Check sheet for the modelled part. Datum: model origin and axes. Units: mm. Round coordinates to 2 decimals unless told otherwise and drop trailing zeros. Write each loop counter-clockwise with the first axis right and the second up, starting at its lowest first coordinate (ties: lowest second). Pieces come first, ordered by that corner, then holes.
Item 1: Cross-section at D-D on x = 32. Enter the section's corners in (y, z).
Item 2: Cross-section at B-B on z = 1.2. Enter the section's corners in (x, y), plus the area to 3 significant figures.
Item 3: Cross-section at C-C on y = 20.5. Count the separate pieces of the cut face and the enclosed holes in it, plus the area to 3 significant figures.
Item 4: Material ranges on line 1 (X direction, y = 23, z = 0.9); line 2 (X direction, y = 7.5, z = 0.9); line 3 (Y direction, x = 23.5, z = 0.95), recorded low to high.
Item 5: Go/stop test with a flat-tipped pin: pin 1 Ø0.5 at (y, z) = (10, 1) entering from +X. Record where the tip stops, or that it passes through.
Item 6: Cross-section at A-A on y = 11. Enter the section's corners in (x, z).
from build123d import *

# Parameters (mm, degrees)
BOSS_EXTRUDE2_DEPTH                       = 186.944
CUT_EXTRUDE1_DEPTH                        = 190.568748947
SKETCH6_W                                 = 6.35
SKETCH6_H                                 = 6.1722
CUT_EXTRUDE3_DEPTH                        = 190.568748947
CSK_FOR_6_FLAT_HEAD_MACHINE_SCREW_2_COUNT = 2
CSK_FOR_6_FLAT_HEAD_MACHINE_SCREW_2_PITCH = 95.25


with BuildPart() as part:
    # Sketch3 → Boss-Extrude2 (new body)
    with BuildSketch(Plane(origin=(0, 0, 0), x_dir=(0, 0, -1), z_dir=(1, 0, 0))):
        Polygon((-0.5715, 31.420044321), (-1.5875, 30.833456448), (-1.5875, -1.917455679), (-0.5715, -1.330867805), align=None)
    extrude(amount=BOSS_EXTRUDE2_DEPTH)

    # Sketch5 → Cut-Extrude1 (cut, through all)
    with BuildSketch(Plane.XY.offset(1.5875)):
        Polygon((0, -1.917455679), (16.672349491, 31.420044321), (0, 31.420044321), align=None)
        Polygon((186.944, -1.917455679), (186.944, 31.420044321), (170.271650509, 31.420044321), align=None)
    extrude(amount=-CUT_EXTRUDE1_DEPTH, mode=Mode.SUBTRACT)

    # Sketch6 → Cut-Extrude3 (cut, through all)
    with BuildSketch(Plane.XY.offset(1.5875)):
        with Locations((22.352, 20.210554054)):
            Rectangle(SKETCH6_W, SKETCH6_H)
        with Locations((46.482, 9.753360379)):
            Rectangle(SKETCH6_W, SKETCH6_H)
        with Locations((141.732, 9.753360379)):
            Rectangle(SKETCH6_W, SKETCH6_H)
        with Locations((165.862, 20.210554054)):
            Rectangle(SKETCH6_W, SKETCH6_H)
    extrude(amount=-CUT_EXTRUDE3_DEPTH, mode=Mode.SUBTRACT)

    # Sketch7 → CSK for #6 Flat Head Machine Screw (100)1 (revolve, cut)
    with BuildSketch(Plane(origin=(46.482, 19.486654054, 1.5875), x_dir=(0, -1, 0), z_dir=(1, 0, 0))):
        Polygon((0, 0), (0, 1.016), (1.89865, 1.016), (1.89865, 1.380025208), (3.5433, 0), align=None)
    csk_for_6_flat_head_machine_screw_100 = revolve(axis=Axis((46.482, 19.486654054, 7.9375), (0, 0, -1)), mode=Mode.SUBTRACT)

    # CSK for _6 Flat Head Machine Screw _ 2: CSK for #6 Flat Head Machine Screw (100)1 ×2
    with Locations(*[(i * CSK_FOR_6_FLAT_HEAD_MACHINE_SCREW_2_PITCH, 0, 0) for i in range(1, CSK_FOR_6_FLAT_HEAD_MACHINE_SCREW_2_COUNT)]):
        add(csk_for_6_flat_head_machine_screw_100, mode=Mode.SUBTRACT)


solid = part.part
Response values:
1. outline: (-1.92, 1.59) - (-1.33, 0.57) - (31.42, 0.57) - (30.83, 1.59) - close
2. outline: (0.11, -1.69) - (186.83, -1.69) - (170.45, 31.06) - (16.49, 31.06) - close; hole (19.18, 17.12) - (25.53, 17.12) - (25.53, 23.3) - (19.18, 23.3) - close; hole (43.31, 6.67) - (49.66, 6.67) - (49.66, 12.84) - (43.31, 12.84) - close; hole circle Ø6.16 at (46.48, 19.49); hole (138.56, 6.67) - (144.91, 6.67) - (144.91, 12.84) - (138.56, 12.84) - close; hole circle Ø6.16 at (141.73, 19.49); hole (162.69, 17.12) - (169.04, 17.12) - (169.04, 23.3) - (162.69, 23.3) - close
2. area: 5,360 mm2
3. separate pieces: 5
3. enclosed holes: 0
3. area: 143 mm2
4. line 1: x = 12.46 to 19.18, 25.53 to 162.69, 169.04 to 174.48
4. line 2: x = 4.71 to 43.31, 49.66 to 138.56, 144.91 to 182.23
4. line 3: y = -1.55 to 17.12, 23.3 to 31.2
5. pin 1: stops at x = 181.11
6. outline: (6.46, 0.57) - (43.31, 0.57) - (43.31, 1.59) - (6.46, 1.59) - close; (49.66, 0.57) - (138.56, 0.57) - (138.56, 1.59) - (49.66, 1.59) - close; (144.91, 0.57) - (180.48, 0.57) - (180.48, 1.59) - (144.91, 1.59) - close
